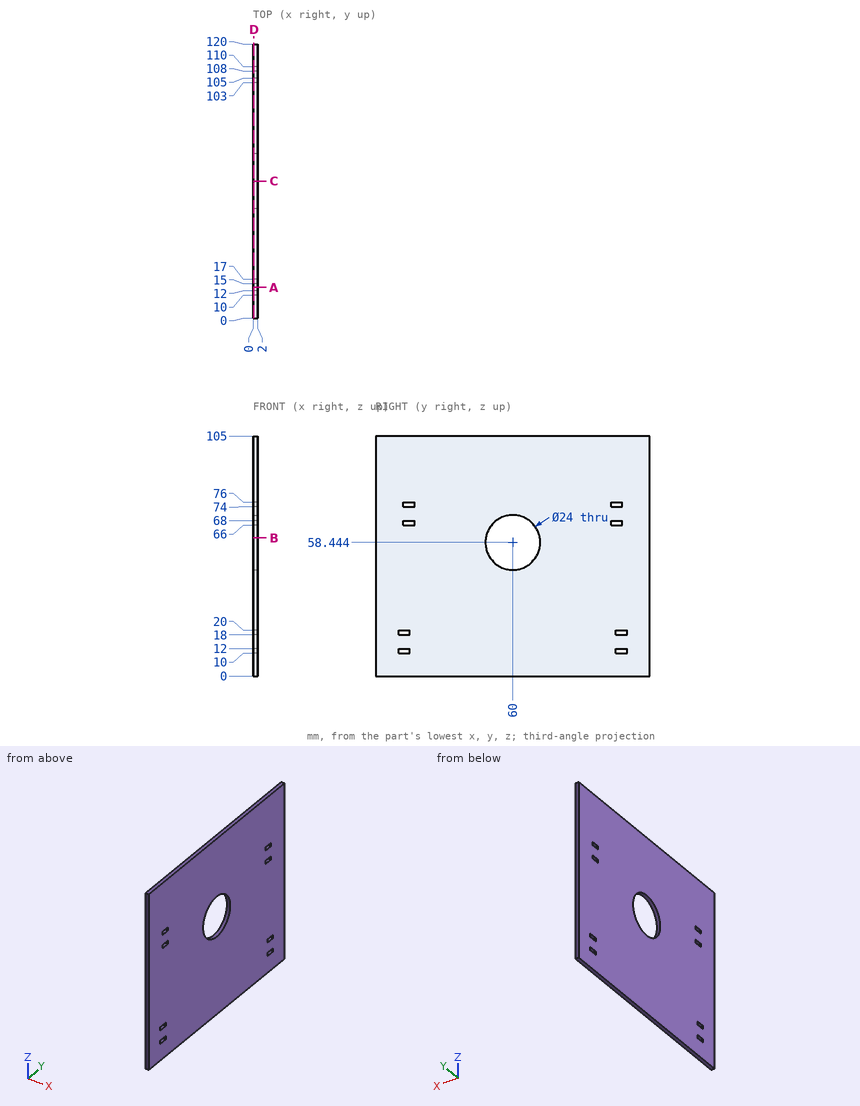
The figure shows three views and two pictorial views of one solid part (mm, origin at its lowest corner). Answer the questions. Round coordinates to 2 decimals unless told otherwise and drop trailing zeros. Write each loop counter-clockwise with the first axis right and the second up, starting at its lowest first coordinate (ties: lowest second). Pieces come first, ordered by that corner, then holes. Notation, with made-up numbers: (1, -37) -> (27, -37) arc R15 cw to (27, -33) -> close; hole circle Ø10 at (23, 47). An arc over 180 degrees is marked (long way). Answer as a JSON object with one key per item and string values. Group by question number.
Q1. Section B-B (z = 60.5) is taken. Write down the section's boundary in (x, y).
Q2. Straight lines are drawn through the part: line 1 along Y through (x, z) = (1.75, 19.5); line 2 along Z through (x, y) = (0.3, 108.5); line 3 along Z through (x, y) = (1.05, 60). For each, find the intervals that lie inside material, in ascending order.
Q3. Section C-C (y = 60) is taken. Write down the section's boundary in (x, z).
Q4. Section D-D (x = 0.35) is taken. Count the separate pieces of the cut face and the enclosed holes in it, plus the area to 3 significant figures.
Q5. Section A-A (y = 13.5) is taken. Write down the section's boundary in (x, z).
Check values:
{
 "1": {"outline": "(0, 0) -> (2, 0) -> (2, 48.18) -> (0, 48.18) -> close; (0, 71.82) -> (2, 71.82) -> (2, 120) -> (0, 120) -> close"},
 "2": {"line 1": "0 to 10, 15 to 105, 110 to 120", "line 2": "0 to 10, 12 to 18, 20 to 105", "line 3": "0 to 46.44, 70.44 to 105"},
 "3": {"outline": "(0, 0) -> (2, 0) -> (2, 46.44) -> (0, 46.44) -> close; (0, 70.44) -> (2, 70.44) -> (2, 105) -> (0, 105) -> close"},
 "4": {"separate pieces": "1", "enclosed holes": "9", "area": "12,100 mm^2"},
 "5": {"outline": "(0, 0) -> (2, 0) -> (2, 10) -> (0, 10) -> close; (0, 12) -> (2, 12) -> (2, 18) -> (0, 18) -> close; (0, 20) -> (2, 20) -> (2, 66) -> (0, 66) -> close; (0, 68) -> (2, 68) -> (2, 74) -> (0, 74) -> close; (0, 76) -> (2, 76) -> (2, 105) -> (0, 105) -> close"}
}
